Geometry check sheet. Reference: the model listing, model coordinates, mm. A direction names the side the tool comes from. Round coordinates to 2 decimals unless told otherwise and drop trailing zeros. Use a Markdown table: item, result.
```python
from build123d import *

# Parameters (mm, degrees)
SKETCH1_R           = 175
SKETCH1_R_2         = 29
BOSS_EXTRUDE1_DEPTH = 7
CUT_EXTRUDE1_START  = -2
SKETCH2_R           = 175
SKETCH2_R_2         = 135
CUT_EXTRUDE1_DEPTH  = 2
SKETCH3_R           = 5
CUT_EXTRUDE2_DEPTH  = 248.586348574
CIRPATTERN1_COUNT   = 3
SKETCH4_R           = 8
CUT_EXTRUDE3_DEPTH  = 1.5
CIRPATTERN2_COUNT   = 3
CUT_EXTRUDE5_START  = -7
CUT_EXTRUDE5_DEPTH  = 7
CIRPATTERN3_COUNT   = 5
SKETCH6_R           = 2.5
CUT_EXTRUDE6_DEPTH  = 248.586348718
CIRPATTERN4_COUNT   = 13
SKETCH8_R           = 175
SKETCH8_R_2         = 135
CUT_EXTRUDE7_DEPTH  = 0.01
SKETCH9_W           = 90.900327039
SKETCH9_H           = 40.914041524
CUT_EXTRUDE8_DEPTH  = 0.001
SKETCH10_W          = 130.294838349
SKETCH10_H          = 54.011108205
CUT_EXTRUDE9_DEPTH  = 0.01
SKETCH11_W          = 108.207821592
SKETCH11_H          = 46.030085343
CUT_EXTRUDE10_DEPTH = 0.01


# Read off the part's stored shape, not the designer's step: Cut-Extrude5
with BuildPart() as part:
    # Sketch1 → Boss-Extrude1 (new body)
    with BuildSketch(Plane.XY):
        Circle(SKETCH1_R)
        Circle(SKETCH1_R_2, mode=Mode.SUBTRACT)
    extrude(amount=BOSS_EXTRUDE1_DEPTH)

    # Sketch2 → Cut-Extrude1 (cut)
    with BuildSketch(Plane.XY.offset(7).offset(CUT_EXTRUDE1_START)):
        Circle(SKETCH2_R)
        Circle(SKETCH2_R_2, mode=Mode.SUBTRACT)
    extrude(amount=CUT_EXTRUDE1_DEPTH, mode=Mode.SUBTRACT)

    # Sketch3 → Cut-Extrude2 (cut, through all)
    with BuildSketch(Plane.XY.offset(7)):
        with Locations((0, 40.8)):
            Circle(SKETCH3_R)
    cut_extrude2 = extrude(amount=-CUT_EXTRUDE2_DEPTH, mode=Mode.SUBTRACT)

    # CirPattern1: Cut-Extrude2 ×3 about axis
    cirpattern1_axis = Axis((0, 0, 0), (0, 0, 1))
    for i in range(1, CIRPATTERN1_COUNT):
        add(cut_extrude2.rotate(cirpattern1_axis, i * 360 / CIRPATTERN1_COUNT), mode=Mode.SUBTRACT)

    # Sketch4 → Cut-Extrude3 (cut)
    with BuildSketch(Plane.XY.offset(7)):
        with Locations((0, 40.8)):
            Circle(SKETCH4_R)
    cut_extrude3 = extrude(amount=-CUT_EXTRUDE3_DEPTH, mode=Mode.SUBTRACT)

    # CirPattern2: Cut-Extrude3 ×3 about axis
    cirpattern2_axis = Axis((0, 0, 0), (0, 0, 1))
    for i in range(1, CIRPATTERN2_COUNT):
        add(cut_extrude3.rotate(cirpattern2_axis, i * 360 / CIRPATTERN2_COUNT), mode=Mode.SUBTRACT)

    # Cut-Extrude5 outline → Cut-Extrude5 (cut)
    with BuildSketch(Plane.XY.offset(7).offset(CUT_EXTRUDE5_START)):
        with BuildLine():
            ThreePointArc((121.499939496, -0.12298749), (124.999939496, -3.62298749), (128.499939496, -0.12298749))
            add(Edge.make_bspline(
                [(128.499939496, -0.12298749), (128.499939496, 31.638419222), (107.348855254, 74.121828628), (52.396465064, 93.291267066), (8.993017656, 92.632641356), (-8.214226951, 71.193884394)],
                knots=[0, 0, 0, 0, 0, 0, 1, 1, 1, 1, 1, 1], degree=5))
            ThreePointArc((-8.214226951, 71.193884394), (-8.426452431, 57.069934817), (5.212663873, 53.394952133))
            add(Edge.make_bspline(
                [(5.212663873, 53.394952133), (27.795809489, 63.896743321), (53.784046438, 66.244067949), (78.598621074, 55.010442945), (99.053878543, 43.441485852), (121.499939496, 28.129262896), (121.499939496, -0.12298749)],
                knots=[0, 0, 0, 0, 0, 0, 0, 1, 1, 1, 1, 1, 1, 1], degree=6))
        make_face()
    cut_extrude5 = extrude(amount=CUT_EXTRUDE5_DEPTH, mode=Mode.SUBTRACT)

    # CirPattern3: Cut-Extrude5 ×5 about axis
    cirpattern3_axis = Axis((0, 0, 7), (0, 0, 1))
    for i in range(1, CIRPATTERN3_COUNT):
        add(cut_extrude5.rotate(cirpattern3_axis, i * 360 / CIRPATTERN3_COUNT), mode=Mode.SUBTRACT)

    # Sketch6 → Cut-Extrude6 (cut, through all)
    with BuildSketch(Plane.XY.offset(7)):
        with Locations((0, 138.943546743)):
            Circle(SKETCH6_R)
        with Locations((9.192388155, 148.135934899)):
            Circle(SKETCH6_R)
        with Locations((18.384776311, 157.328323054)):
            Circle(SKETCH6_R)
        with Locations((27.577164466, 166.520711209)):
            Circle(SKETCH6_R)
    cut_extrude6 = extrude(amount=-CUT_EXTRUDE6_DEPTH, mode=Mode.SUBTRACT)

    # CirPattern4: Cut-Extrude6 ×13 about axis
    cirpattern4_axis = Axis((0, 0, 0), (0, 0, 1))
    for i in range(1, CIRPATTERN4_COUNT):
        add(cut_extrude6.rotate(cirpattern4_axis, i * 360 / CIRPATTERN4_COUNT), mode=Mode.SUBTRACT)

    # Sketch8 → Cut-Extrude7 (cut)
    with BuildSketch(Plane.XY):
        Circle(SKETCH8_R)
        Circle(SKETCH8_R_2, mode=Mode.SUBTRACT)
    extrude(amount=CUT_EXTRUDE7_DEPTH, mode=Mode.SUBTRACT)

    # Sketch9 → Cut-Extrude8 (cut)
    with BuildSketch(Plane.XY):
        with Locations((4.527748237, 155.446859957)):
            Rectangle(SKETCH9_W, SKETCH9_H)
    extrude(amount=CUT_EXTRUDE8_DEPTH, mode=Mode.SUBTRACT)

    # Sketch10 → Cut-Extrude9 (cut)
    with BuildSketch(Plane.XY.offset(5)):
        with Locations((4.215957898, 161.982952097)):
            Rectangle(SKETCH10_W, SKETCH10_H)
    extrude(amount=-CUT_EXTRUDE9_DEPTH, mode=Mode.SUBTRACT)

    # Sketch11 → Cut-Extrude10 (cut)
    with BuildSketch(Plane(origin=(0, 0, 0.01), x_dir=(-1, 0, 0), z_dir=(0, 0, -1))):
        with Locations((-1.268876231, 158.398747535)):
            Rectangle(SKETCH11_W, SKETCH11_H)
    extrude(amount=-CUT_EXTRUDE10_DEPTH, mode=Mode.SUBTRACT)


solid = part.part
```
Item 1: Go/stop test with flat-tipped pins: pin 1 (3 mm diameter, centred on x = -119.03, y = 104.5, fed in from +Z); pin 2 (6.5 mm diameter, centred on x = 101.8, y = 134.63, fed in from -Z); pin 3 (3 mm diameter, centred on y = -82.5, z = 3.5, fed in from +X). Record where each tip stops, or that it passes through.
Outcome:
| item | result |
|---|---|
| pin 1 | passes through |
| pin 2 | stops at z = 0.01 |
| pin 3 | stops at x = 155.13 |
Item 2: Mould release check, pull along X, two halves, no side actions. Record for faces 4 (the face through (-1.041, 48.732, 6.26)), 5 (the face through (-32, 2, 7)), 6 (the face through (-128.982, 118.273, 2.47)): +X half, -X half, draft (parallel to the pull), parting line (faces both ways), or undercut.
Outcome:
| item | result |
|---|---|
| face 4 | undercut |
| face 5 | draft |
| face 6 | parting line |
Item 3: Cross-section at A-A, the plane y = -20.4. Count the separate pieces of the cut face and the enclosed holes in it, and give its area (3 significant figures).
Outcome:
| item | result |
|---|---|
| separate pieces | 6 |
| enclosed holes | 0 |
| area | 1,470 mm2 |
Item 4: Access from +Z, -Z, +X, -X, +Y, -Y to the whole of each face (thin tool, end or side, straight path). Record for faces 1 (the face through (-57.083, 9.554, 3.451)), 2 (the face through (-30.8, -17.9, 5.5)), 3 (the face through (2, 155, 0.02)).
Outcome:
| item | result |
|---|---|
| face 1 | +Z, -Z |
| face 2 | +Z |
| face 3 | -Z, +X, -X, +Y, -Y |
Item 5: Material ranges on line 1 along X through (y, z) = (48.5, 1.5); line 2 along Y through (x, z) = (-11.5, 6); line 3 along Y through (x, z) = (-22, 5.75), recorded low to high. Write a range as from..to.
Outcome:
| item | result |
|---|---|
| line 1 | x = -168.15..-164.25, -159.71..-115.46, -106.1..-73.56, -47.8..84.39, 108.97..168.15 |
| line 2 | y = -134.51..-102.81, -80.9..-26.62, 26.62..102.7, 119.02..134.51 |
| line 3 | y = -133.2..-104.75, -84.83..-18.89, 18.89..93.31, 113.93..133.2 |
